Build history of the part. All positions in model axes, mm. Face numbers are marked on the shaded views. Round coordinates to 2 decimals unless told otherwise and drop trailing zeros. Order: outer loops, then holes, each group sorted by start corner. A loop starts at its lowest first (then second) coordinate and runs counter-clockwise, first axis right, second up. Notation, with made-up numbers: M -38.75,73.25 L 4.25,73.25 A16 ccw 4.25,99.25 Z; hole C -3.5,88.25 d9. An arc over 180 degrees is marked long. Use CSV: the item, a comma, the result in double quotes.
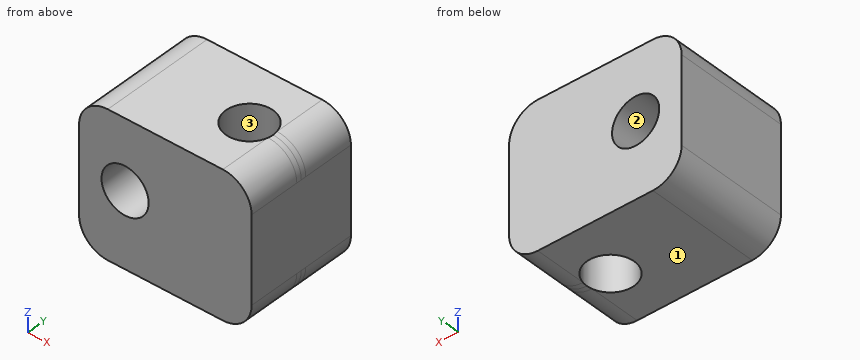
from build123d import *

# Parameters (mm, degrees)
SKETCH_1_W          = 30
SKETCH_1_H          = 20
EXTRUDE_1_DEPTH     = 25
SKETCH_2_R          = 4.1
CUT_EXTRUDE_1_DEPTH = 25
SKETCH_3_R          = 4.1
CUT_EXTRUDE_2_DEPTH = 25
FILLET_2_R          = 5


with BuildPart() as part:
    # 草图1 → 凸台-拉伸1 (new body)
    with BuildSketch(Plane.XY):
        Rectangle(SKETCH_1_W, SKETCH_1_H)
    extrude(amount=EXTRUDE_1_DEPTH)

    # 草图2 → 切除-拉伸1 (cut)
    with BuildSketch(Plane.XY.offset(25)):
        with Locations((6, 0)):
            Circle(SKETCH_2_R)
    extrude(amount=-CUT_EXTRUDE_1_DEPTH, mode=Mode.SUBTRACT)

    # 草图3 → 切除-拉伸2 (cut)
    with BuildSketch(Plane(origin=(0, 10, 0), x_dir=(1, 0, 0), z_dir=(0, 1, 0))):
        with Locations(Location((-7, -13, 0), (0, 0, 270))):
            Circle(SKETCH_3_R)
    extrude(amount=-CUT_EXTRUDE_2_DEPTH, mode=Mode.SUBTRACT)

    # 圆角2
    fillet_2_edges = [part.edges().sort_by_distance(p)[0] for p in [
        (-15, 0, 25),
        (15, 0, 25),
        (-15, 0, 0),
        (15, 0, 0),
    ]]
    fillet(fillet_2_edges, radius=FILLET_2_R)


solid = part.part
(1) Wall check: line 1 (X direction, y = -1, z = 16); line 2 (X direction, y = 2.25, z = 13); line 3 (X direction, y = 0, z = 7.5). Give the ranges that are in metal, low to high. Write a range as from..to.
Answer block:
line 1,"x = -15..-9.79, -4.21..2.02, 9.98..15"
line 2,"x = -15..-11.1, -2.9..2.57, 9.43..15"
line 3,"x = -15..1.9, 10.1..15"
(2) Cut at B-B, the plane z = 13. Give the cut face in (x, y).
Answer block:
outline,"M -15,-10 L -11.1,-10 L -11.1,10 L -15,10 Z; M -2.9,-10 L 15,-10 L 15,10 L -2.9,10 Z; hole C 6,0 d8.2"
(3) Cut at D-D, the plane z = 6.75. Give the cut face in (x, y), and give its area (3 significant figures).
Answer block:
outline,"M -15,-10 L 15,-10 L 15,10 L -15,10 Z; hole C 6,0 d8.2"
area,"547 mm²"
(4) Drop flat-ended pins along their axis: pin 1 (10.5 mm diameter, centred on x = -7, z = 13, fed in from +Y); pin 2 (7.5 mm diameter, centred on x = 6, y = 0, fed in from -Z). Give the stop position or say it passes through.
Answer block:
pin 1,"stops at y = 10"
pin 2,"passes through"
(5) Cut at C-C, the plane y = 9. Give the cut face in (x, z).
Answer block:
outline,"M -15,5 A5 ccw -10,0 L 10,0 A5 ccw 15,5 L 15,20 A5 ccw 10,25 L -10,25 A5 ccw -15,20 Z; hole C -7,13 d8.2"
(6) Two-plate mould, pull along Z, no slides. Class the marked faces 1, 2 and 3: released by +Z, released by -Z, zero draft, split by the parting line, or undercut.
Answer block:
face 1,"released by -Z"
face 2,"undercut"
face 3,"zero draft"
(7) Cut at A-A, the plane x = 6. Give the cut face in (y, z), and give its area (3 significant figures).
Answer block:
outline,"M -10,0 L -4.1,0 L -4.1,25 L -10,25 Z; M 4.1,0 L 10,0 L 10,25 L 4.1,25 Z"
area,"295 mm²"
